```python
from build123d import *

# Parameters (mm, degrees)
SKETCH1_W           = 38
SKETCH1_H           = 38
BOSS_EXTRUDE1_DEPTH = 1.5
SKETCH2_R           = 17.5
BOSS_EXTRUDE2_DEPTH = 10
SKETCH3_R           = 14
BOSS_EXTRUDE3_DEPTH = 40.5
SKETCH4_R           = 12.5
CUT_EXTRUDE1_DEPTH  = 3
SKETCH5_R           = 1.478595514
BOSS_EXTRUDE4_DEPTH = 20
SKETCH6_W           = 22
SKETCH6_H           = 1.5
BOSS_EXTRUDE5_DEPTH = 20


with BuildPart() as part:
    # Sketch1 → Boss-Extrude1 (new body)
    with BuildSketch(Plane(origin=(0, 0, 0), x_dir=(1, 0, 0), z_dir=(0, 1, 0))):
        Rectangle(SKETCH1_W, SKETCH1_H)
    extrude(amount=BOSS_EXTRUDE1_DEPTH)

    # Sketch2 → Boss-Extrude2 (add)
    with BuildSketch(Plane(origin=(0, 1.5, 0), x_dir=(1, 0, 0), z_dir=(0, 1, 0))):
        Circle(SKETCH2_R)
    extrude(amount=BOSS_EXTRUDE2_DEPTH)

    # Sketch3 → Boss-Extrude3 (add)
    with BuildSketch(Plane(origin=(0, 11.5, 0), x_dir=(1, 0, 0), z_dir=(0, 1, 0))):
        Circle(SKETCH3_R)
    extrude(amount=BOSS_EXTRUDE3_DEPTH)

    # Sketch4 → Cut-Extrude1 (cut)
    with BuildSketch(Plane(origin=(0, 52, 0), x_dir=(1, 0, 0), z_dir=(0, 1, 0))):
        Circle(SKETCH4_R)
    extrude(amount=-CUT_EXTRUDE1_DEPTH, mode=Mode.SUBTRACT)

    # Sketch5 → Boss-Extrude4 (add)
    with BuildSketch(Plane(origin=(0, 0, 0), x_dir=(0, 0, -1), z_dir=(1, 0, 0))):
        with Locations((0, 32.23)):
            Circle(SKETCH5_R)
    extrude(amount=BOSS_EXTRUDE4_DEPTH)

    # Sketch6 → Boss-Extrude5 (add)
    with BuildSketch(Plane.XY.offset(19)):
        with Locations((0, 0.75)):
            Rectangle(SKETCH6_W, SKETCH6_H)
    extrude(amount=BOSS_EXTRUDE5_DEPTH)


solid = part.part
```
Input: part model. Units: mm. Frame: model coordinates. A direction names the side the tool comes from. Coordinates: 2 decimals unless noted, no trailing zeros. Loops run counter-clockwise (first coordinate to the right, second up) from the corner with the lowest first, then second, coordinate; pieces in that order, holes last. Notation, with made-up numbers: (50.5, 38.5) -> (61.5, 38.5) arc R23 cw to (61.5, 59.5) -> close; hole circle Ø6 at (80, 76.5). An arc over 180 degrees is marked (long way). Use a Markdown table: item, result.
1) Cut plane D-D (x = 9). Return the cut outline in (y, z), then the cut area to 3 significant figures.
Results found:
| item | result |
|---|---|
| outline | (0, -19) -> (1.5, -19) -> (1.5, -15.01) -> (11.5, -15.01) -> (11.5, -10.72) -> (52, -10.72) -> (52, -8.67) -> (49, -8.67) -> (49, 8.67) -> (52, 8.67) -> (52, 10.72) -> (11.5, 10.72) -> (11.5, 15.01) -> (1.5, 15.01) -> (1.5, 39) -> (0, 39) -> close |
| area | 1,200 mm2 |
2) Access query for faces 5 (the cylindrical face through (11.923, 50.521, -3.755)), 6 (the flat face through (0, 1, -19)), 7 (the flat face through (-19, 1, 0)), 8 (the flat face through (15, 1, 19)), 9 (the flat face through (-11, 1, 29)). Directions: +Z, -Z, +X, -X, +Y, -Y. A direction counts if a zero-diameter tool reaches every point of the face in a straight line with its end or side. Return the directions, or none.
Results found:
| item | result |
|---|---|
| face 5 | +Y |
| face 6 | -Z, +X, -X, +Y, -Y |
| face 7 | +Z, -Z, -X, +Y, -Y |
| face 8 | +Z, +X, +Y, -Y |
| face 9 | +Z, -X, +Y, -Y |
3) Cut plane A-A (x = 0). Return the cut outline in (y, z), then the cut area to 3 significant figures.
Results found:
| item | result |
|---|---|
| outline | (0, -19) -> (1.5, -19) -> (1.5, -17.5) -> (11.5, -17.5) -> (11.5, -14) -> (52, -14) -> (52, -12.5) -> (49, -12.5) -> (49, 12.5) -> (52, 12.5) -> (52, 14) -> (11.5, 14) -> (11.5, 17.5) -> (1.5, 17.5) -> (1.5, 39) -> (0, 39) -> close |
| area | 1,500 mm2 |
4) Material intervals for line 1 along Z through (x, y) = (0, 49.7); line 2 along Y through (x, z) = (-2, -1.5), sorted ascending. Write a range as from..to.
Results found:
| item | result |
|---|---|
| line 1 | z = -14..-12.5, 12.5..14 |
| line 2 | y = 0..49 |
5) Cut plane B-B (z = 0). Return the cut outline in (x, y), then the cut area to 3 significant figures.
Results found:
| item | result |
|---|---|
| outline | (-19, 0) -> (19, 0) -> (19, 1.5) -> (17.5, 1.5) -> (17.5, 11.5) -> (14, 11.5) -> (14, 30.75) -> (20, 30.75) -> (20, 33.71) -> (14, 33.71) -> (14, 52) -> (12.5, 52) -> (12.5, 49) -> (-12.5, 49) -> (-12.5, 52) -> (-14, 52) -> (-14, 11.5) -> (-17.5, 11.5) -> (-17.5, 1.5) -> (-19, 1.5) -> close |
| area | 1,480 mm2 |
6) Pull-direction query (Y, two-part tool) for faces 1 (the flat face through (11, 1, 29)), 2 (the cylindrical face through (16.918, 30.787, 0.321)), 3 (the flat face through (0, 0, 3)), 4 (the flat face through (0, 49, 0)); classes: released by +Y, released by -Y, zero draft, split by the parting line, or undercut.
Results found:
| item | result |
|---|---|
| face 1 | zero draft |
| face 2 | undercut |
| face 3 | released by -Y |
| face 4 | released by +Y |
7) Contact query for flat-ended pins moving along their axis: pin 1 (3 mm diameter, centred on y = 33.5, z = -4.5, fed in from -X); pin 2 (5 mm diameter, centred on x = -6, y = 30, fed in from -Z); pin 3 (12.5 mm diameter, centred on x = 1, z = 1.5, fed in from +Y). Output: stop coordinate, or through.
Results found:
| item | result |
|---|---|
| pin 1 | stops at x = -13.67 |
| pin 2 | stops at z = -13.56 |
| pin 3 | stops at y = 49 |
8) Cut plane C-C (y = 19). Return the cut outline in (x, z).
Results found:
| item | result |
|---|---|
| outline | circle Ø28 at (0, 0) |
